Verification items for the finished model (mm, model axes). A direction names the side the tool comes from. Round coordinates to 2 decimals unless told otherwise and drop trailing zeros. Loops run counter-clockwise (first coordinate to the right, second up) from the corner with the lowest first, then second, coordinate; pieces in that order, holes last. Notation, with made-up numbers: (33, 44.5) - (66, 44.5) arc R24 cw to (66, 65.5) - close; hole circle Ø8 at (-29, 40). An arc over 180 degrees is marked (long way). Use a Markdown table: item, result. Add a question column.
```python
from build123d import *


with BuildPart() as part:
    # Sketch3 → Revolve1 (revolve)
    with BuildSketch(Plane.XY):
        with BuildLine():
            Line((0, 0), (37.465, 0))
            Line((37.465, 0), (37.465, 190.5))
            ThreePointArc((37.465, 190.5), (34.032849621, 205.925272777), (24.384, 218.44))
            Line((24.384, 218.44), (24.384, 250.19))
            Line((24.384, 250.19), (21.209, 250.19))
            Line((21.209, 250.19), (21.209, 218.44))
            ThreePointArc((21.209, 218.44), (31.341590564, 204.463946967), (34.925, 187.577306486))
            Line((34.925, 187.577306486), (34.925, 3.175))
            Line((34.925, 3.175), (0, 3.175))
            Line((0, 3.175), (0, 0))
        make_face()
    revolve(axis=Axis((0, 0, 0), (0, 1, 0)))


solid = part.part
```
Q1. Set-up check for faces 4 (the face through (20.23, 234.09, -6.37)), 5 (the face through (0, 3.175, 0)), 6 (the face through (0, 250.19, -22)): record each of +Z, -Z, +X, -X, +Y, -Y from which the full face is reachable in a straight line by a thin tool's end or side.
Q2. Section check A-A on y = 169. Record the cut outline in (x, z) (3 decimals), plus the area to 3 significant figures.
Q3. Thickness scan on line 1 along X through (y, z) = (72.5, 0) (3 decimals); line 2 along Z through (x, y) = (0, 235). Record the ranges inside material, lowest first.
Q4. Go/stop test with flat-tipped pins: pin 1 Ø1.5 at (y, z) = (25.5, 14) entering from -X; pin 2 Ø6 at (y, z) = (152.5, 5.5) entering from +X; pin 3 Ø3 at (y, z) = (174.5, -8) entering from -X. Record where each tip stops, or that it passes through.
Q5. Release check for a two-part mould opening along Z. For faces 1 (the face through (-27.715, 94.085, 21.251)), 2 (the face through (1, 0, -1)), 3 (the face through (-29.73, 96.58, 22.8)) record: +Z half, -Z half, draft (parallel to the pull), parting line (faces both ways), or undercut.
Determined:
| question | item | result |
|---|---|---|
| 1 | face 4 | +Y |
| 1 | face 5 | none |
| 1 | face 6 | +Z, -Z, +X, -X, +Y |
| 2 | outline | circle Ø74.93 at (0, 0); hole circle Ø69.85 at (0, 0) |
| 2 | area | 578 mm² |
| 3 | line 1 | x = -37.465 to -34.925, 34.925 to 37.465 |
| 3 | line 2 | z = -24.38 to -21.21, 21.21 to 24.38 |
| 4 | pin 1 | stops at x = -35.04 |
| 4 | pin 2 | stops at x = 37.38 |
| 4 | pin 3 | stops at x = -36.9 |
| 5 | face 1 | undercut |
| 5 | face 2 | draft |
| 5 | face 3 | parting line |
